Autodesk Inventor part; units mm, degrees
ref_plane "Work Plane1" through (1.525, 0, 0) normal (0, 0, 1) x (1, 0, 0)
ref_plane "YZ Plane" through (0, 0, 0) normal (1, 0, 0) x (0, 1, 0)
ref_plane "XZ Plane" through (0, 0, 0) normal (0, 1, 0) x (-1, 0, 0)
sketch "Sketch1" plane through (0, 0, 0) normal (0, 0, 1) x (1, 0, 0)
  line L0 (0, 3) -> (38, 3)
  line L1 (38, 3) -> (38, 0)
  line L2 (38, 0) -> (0, 0)
  line L3 (-7.6, 0) -> (45.6, 0)
  line L4 (0, -0.6) -> (0, 3.6)
  line L5 (0, 3) -> (0, 0)
  dimension "d2" = 6
  dimension "d59" = 38
revolve "Body" add sketch "Sketch1" angle 360 about axis through (38, 0, 0) along (-1, 0, 0)
sketch "Sketch2" plane through (0, 0, 0) normal (-1, 0, 0) x (0, 0, 1)
  line L0 (0, 5.1962) -> (4.5, 2.5981)
  line L1 (4.5, 2.5981) -> (4.5, -2.5981)
  line L2 (4.5, -2.5981) -> (0, -5.1962)
  line L3 (0, -5.1962) -> (-4.5, -2.5981)
  line L4 (-4.5, -2.5981) -> (-4.5, 2.5981)
  line L5 (-4.5, 2.5981) -> (0, 5.1962)
  line L6 (-6.3, 0) -> (6.3, 0)
  line L7 (0, 7.2746) -> (0, -7.2746)
  point P0 (0, 0)
  point P1 (0, 0)
  dimension "d11" = 9
extrude "Head" add sketch "Sketch2" along normal blind 4
sketch "Sketch4" plane through (0, 0, 0) normal (0, 0, 1) x (1, 0, 0)
  line L0 (-3.4804, 5.4) -> (-4, 4.5)
  line L1 (-1.1, 0) -> (-0.234, 0)
  line L2 (-4.7532, 0) -> (0.5192, 0)
  line L3 (-4, 5.4) -> (-3.4804, 5.4)
  line L4 (-4, 4.5) -> (-4, 5.4)
  line L5 (0, 6.48) -> (0, -1.08)
  dimension "d65" = 9
  dimension "d67" = 30
  dimension "d68" = 10.8
  dimension "d69" = 4
revolve "Chamfer1" cut sketch "Sketch4" angle 360 about axis through (-1.1, 0, 0) along (1, 0, 0)
thread "Thread"
chamfer "Chamfer2" distance 0.6135 distance2 0.6136 1 edges at (38, -3, 0) measured on face at (38, 0.7485, -0.9828)
fillet "Fillet2" radius 0.3 1 edges at (0, -3, 0)
ref_plane "Work Plane1" through (1.525, 0, 0) normal (0, 0, 1) x (1, 0, 0)
equation "\"d71\" = RR"
equation "\"d11\" = SW"
equation "\"d3\" = KOH"
equation "\"d15\" = GEL"
equation "\"d6\" = -0.5 * SPD + 0.5 * GD"
equation "\"d2\" = GD"
equation "\"d59\" = NLG"
equation "\"d65\" = SW"
equation "\"d67\" = ANG1"
equation "\"d68\" = 1.2 * SW"
equation "\"d69\" = KOH"
equation "\"NLG\" = 38"
equation "\"GD\" = NND"
equation "\"BDM\" = NND"
equation "\"KOH\" = 4"
equation "\"GEL\" = 11"
equation "\"SW\" = 9"
equation "\"SW0\" = SW"
equation "\"SPD\" = NND - 1.2269 * PTC"
equation "\"SD2\" = NND"
equation "\"SD\" = 0"
equation "\"ANG1\" = 30deg"
equation "\"GAL\" = 0.61345 * PTC"
equation "\"GUL\" = 0.61345 * PTC"
equation "\"RR\" = 0.3"
equation "\"RR1\" = 0.1"
equation "\"GD1\" = THREADDIA - 1.2269 * PTC"
equation "\"THREADDIA\" = 6"
equation "\"TOA\" = 30deg"
equation "\"FAWI\" = 60deg"
equation "\"PTC\" = 1"
equation "\"NND\" = 6"
equation "\"E0\" = 1.155 * SW"
properties part number "STN 02 1201 - M6 x 38" material "Steel, Mild"
Geometry check sheet. Reference: the model listing, model coordinates, mm. A direction names the side the tool comes from. Coordinates: 2 decimals unless noted, no trailing zeros. Loops run counter-clockwise (first coordinate to the right, second up) from the corner with the lowest first, then second, coordinate; pieces in that order, holes last. Notation, with made-up numbers: (63, 58.5) - (101, 58.5) arc R25 ccw to (101, 72.5) - close; hole circle Ø3 at (41.25, 16). An arc over 180 degrees is marked (long way). One line per item, written item: value. Start each with the question number.
(1) Tool access check on faces 1 (the flat face through (-1.972, -3.915, -2.219)), 2 (the flat face through (0, -3.4, -1.1)). Record the directions out of +Z, -Z, +X, -X, +Y, -Y that give a thin tool (end or side, any length) a straight path to the whole face; none if there is none.
(2) Cross-section at A-A on x = 25. Enter the section's corners in (y, z).
(3) Depth check by flat-ended pin: P1, Ø5, axis at x = 24, z = -0.5, coming from the -Y side; P2, Ø5, axis at x = 27, z = -1, coming from the +Y side; P3, Ø1.5, axis at x = 2.5, y = -0.5, coming from the +Z side; P4, Ø2.5, axis at y = 2.5, z = 0.5, coming from the +X side. Enter the tip coordinate at first touch or a pass-through.
(4) Material ranges on line 1 (X direction, y = -2.25, z = -2.75); line 2 (Y direction, x = 3.5, z = 0); line 3 (Z direction, x = 23, y = -1.5), recorded low to high. Write a range as [from, to].
Results below:
1. face 1: -Z, +X, -X, -Y
1. face 2: +X
2. outline: circle Ø6 at (0, 0)
3. P1: stops at y = -3
3. P2: stops at y = 3
3. P3: stops at z = 3
3. P4: stops at x = 38
4. line 1: x = [-4, 0]
4. line 2: y = [-3, 3]
4. line 3: z = [-2.6, 2.6]
